```python
from build123d import *

# Parameters (mm, degrees)
BOSS_EXTRUDE1_DEPTH      = 25
BOSS_EXTRUDE1_DEPTH_BACK = 25
BOSS_EXTRUDE2_DEPTH      = 15
BOSS_EXTRUDE2_DEPTH_BACK = 25
SKETCH2_R                = 15
CUT_EXTRUDE1_DEPTH       = 101.069975517
CUT_EXTRUDE2_DEPTH       = 93.466210045
CUT_EXTRUDE3_DEPTH       = 93.466210045
CUT_EXTRUDE4_DEPTH       = 6


with BuildPart() as part:
    # Sketch1 → Boss-Extrude1 (new, two sides: drawn at the far end of the back side and taken through both)
    with BuildSketch(Plane.XY.offset(-BOSS_EXTRUDE1_DEPTH_BACK)):
        Polygon((-14.682422452, 0), (0, 0), (0, 10.443131462), (0, 70), (-12, 70), (-12, 32), (-12, 12), (-55, 12), (-67, 12), (-67, 0), align=None)
    extrude(amount=BOSS_EXTRUDE1_DEPTH + BOSS_EXTRUDE1_DEPTH_BACK)

    # Sketch1_3 → Boss-Extrude2 (add, two sides: drawn at the far end of the back side and taken through both)
    with BuildSketch(Plane.XY.offset(-BOSS_EXTRUDE2_DEPTH_BACK)):
        with BuildLine():
            Line((-55, 32), (-55, 12))
            Line((-55, 12), (-12, 12))
            Line((-12, 12), (-12, 32))
            Line((-12, 32), (-29, 32))
            Line((-29, 32), (-29, 28.000000026))
            ThreePointArc((-29, 28.000000026), (-23, 22.000000026), (-29, 16.000000026))
            Line((-29, 16.000000026), (-37.999206574, 16.000000026))
            ThreePointArc((-37.999206574, 16.000000026), (-44.000000013, 21.999603287), (-38, 28.000000026))
            Line((-38, 28.000000026), (-38, 32))
            Line((-38, 32), (-55, 32))
        make_face()
    extrude(amount=BOSS_EXTRUDE2_DEPTH + BOSS_EXTRUDE2_DEPTH_BACK)

    # Sketch2 → Cut-Extrude1 (cut, through all)
    with BuildSketch(Plane.XZ):
        with Locations((-67, 0)):
            Circle(SKETCH2_R)
    extrude(amount=-CUT_EXTRUDE1_DEPTH, mode=Mode.SUBTRACT)

    # Sketch3 → Cut-Extrude2 (cut, through all)
    with BuildSketch(Plane.ZY.offset(12)):
        with BuildLine():
            ThreePointArc((-25, 45), (-20.615528128, 59.142135624), (-9, 68.323807579))
            ThreePointArc((-9, 68.323807579), (-4.577379737, 69.577379737), (0, 70))
            Line((0, 70), (-25, 70))
            Line((-25, 70), (-25, 45))
        make_face()
        with BuildLine():
            Line((25, 70), (0, 70))
            ThreePointArc((0, 70), (17.67766953, 62.67766953), (25, 45))
            Line((25, 45), (25, 70))
        make_face()
    extrude(amount=-CUT_EXTRUDE2_DEPTH, mode=Mode.SUBTRACT)

    # Sketch3_6 → Cut-Extrude3 (cut, through all)
    with BuildSketch(Plane.ZY.offset(12)):
        with BuildLine():
            ThreePointArc((9, 45), (0, 54), (-9, 45))
            Line((-9, 45), (9, 45))
        make_face()
        with BuildLine():
            Line((9, 45), (-9, 45))
            ThreePointArc((-9, 45), (-6.363961031, 38.636038969), (0, 36))
            ThreePointArc((0, 36), (6.363961031, 38.636038969), (9, 45))
        make_face()
    extrude(amount=-CUT_EXTRUDE3_DEPTH, mode=Mode.SUBTRACT)

    # Sketch3_7 → Cut-Extrude4 (cut)
    with BuildSketch(Plane.ZY.offset(12)):
        with BuildLine():
            Line((-9, 68.323807579), (-9, 45))
            ThreePointArc((-9, 45), (6.363961031, 51.363961031), (0, 36))
            Line((0, 36), (25, 36))
            Line((25, 36), (25, 45))
            ThreePointArc((25, 45), (14.142135624, 65.615528128), (-9, 68.323807579))
        make_face()
    extrude(amount=-CUT_EXTRUDE4_DEPTH, mode=Mode.SUBTRACT)


solid = part.part
```
Can you work these out from the model? Positions are in its coordinate system, mm. A direction names the side the tool comes from. Round coordinates to 2 decimals unless told otherwise and drop trailing zeros. Loops run counter-clockwise (first coordinate to the right, second up) from the corner with the lowest first, then second, coordinate; pieces in that order, holes last. Notation, with made-up numbers: M 43.25,76.5 L 65.25,76.5 A20 cw 65.25,111.5 Z; hole C 31.25,12.5 d6. An arc over 180 degrees is marked long. Answer in a Markdown table with one row per item.
1. If we section it at D-D, the plane y = 65: Please give me the cut outline in (x, z), plus the area to 3 significant figures.
Established:
| item | result |
|---|---|
| outline | M -12,-15 L 0,-15 L 0,15 L -6,15 L -6,-9 L -12,-9 Z |
| area | 216 mm² |
2. If we section it at A-A, the plane y = 22: Please give me the cut outline in (x, z).
Established:
| item | result |
|---|---|
| outline | M -55,-25 L -44,-25 L -44,15 L -55,15 L -55,9 A15 cw -55,-9 Z; M -23,-25 L 0,-25 L 0,25 L -12,25 L -12,15 L -23,15 Z |
3. If we section it at B-B, the plane z = -6: Please give me the cut outline in (x, y).
Established:
| item | result |
|---|---|
| outline | M -53.25,0 L 0,0 L 0,38.29 L -12,38.29 L -12,32 L -29,32 L -29,28 A6 cw -29,16 L -38,16 A6 cw -38,28 L -38,32 L -53.25,32 Z; M -6,51.71 L 0,51.71 L 0,69.27 L -6,69.27 Z |
4. Thinking about a two-plate mould opening in X: for faces 1 (the face through (-9, 57, -9)), 2 (the face through (0, 35, 0)), 3 (the face through (-33, 16, -5)), 4 (the face through (-55, 22, -17)), which applies, pulls with the +X half, pulls with the -X half, needs draft (parallel to the pull), parting line crosses it, or undercut?
Established:
| item | result |
|---|---|
| face 1 | needs draft |
| face 2 | pulls with the +X half |
| face 3 | undercut |
| face 4 | pulls with the -X half |
5. I'm going to push flat-ended pins straight in: pin 1 Ø5 at (y, z) = (20, 12) entering from -X; pin 2 Ø2 at (y, z) = (29, 4.5) entering from -X; pin 3 Ø6 at (x, z) = (-59.5, -19.5) entering from +Y. Where does each tip first touch, or does it pass through?
Established:
| item | result |
|---|---|
| pin 1 | x = -55 |
| pin 2 | x = -53.04 |
| pin 3 | y = 12 |
6. Please list where these lines run through material, in increasing order: line 1 (Y direction, x = -20, z = -18.5); line 2 (X direction, y = 53.5, z = -13); line 3 (X direction, y = 31, z = -12). Write a range as from..to.
Established:
| item | result |
|---|---|
| line 1 | 0..32 |
| line 2 | -12..0 |
| line 3 | -55..-38, -29..0 |
7. On a 3-axis mill with a long thin cutter (end or side, diameter ignored), from which of +Z, -Z, +X, -X, +Y, -Y can I reach the whole of each face in a straight line? I mean faces 5 (the face through (-27, 8, 25)), 6 (the face through (-6, 53, 8)), 7 (the face through (-20, 32, -5)), 8 (the face through (-34, 0, 0)), 9 (the face through (-38, 30, -5)). Say none if no direction works.
Established:
| item | result |
|---|---|
| face 5 | +Z, +X, -X, +Y, -Y |
| face 6 | +Z, -X, +Y |
| face 7 | +Z, -Z, -X, +Y |
| face 8 | +Z, -Z, +X, -X, -Y |
| face 9 | +Z, -Z, +Y |
8. If we section it at C-C, the plane x = -39: Please give me the cut outline in (y, z).
Established:
| item | result |
|---|---|
| outline | M 0,-25 L 16.08,-25 L 16.08,15 L 12,15 L 12,25 L 0,25 Z; M 27.92,-25 L 32,-25 L 32,15 L 27.92,15 Z |
